from build123d import *

# Parameters (mm, degrees)
F0_W     = 152.4
F0_H     = 25.019
F0_H_2   = 0.762
F1_DEPTH = 9.525
F2_DEPTH = 2.032
F4_DEPTH = 3.175
F5_DEPTH = 9.525
F6_DEPTH = 9.525


with BuildPart() as f1:
    # F0 (on Top) → F1 (new body)
    with BuildSketch(Plane.XY):
        with Locations((35.9758849268, -12.9505327462)):
            Rectangle(F0_W, F0_H)
        with Locations((35.9758849268, 12.8304672538)):
            Rectangle(F0_W, F0_H)
        with Locations((35.9758849268, -0.0600327462)):
            Rectangle(F0_W, F0_H_2)
    extrude(amount=-F1_DEPTH)

    # F0 (on Top) → F2 (cut)
    with BuildSketch(Plane.XY):
        with Locations((35.9758849268, -0.0600327462)):
            Rectangle(F0_W, F0_H_2)
    extrude(amount=-F2_DEPTH, mode=Mode.SUBTRACT)

    # F3 (on face) → F4 (cut)
    with BuildSketch(Plane.XY):
        with BuildLine():
            Line((-30.6991150732, 18.6724672538), (-30.6991150732, 5.9724672538))
            ThreePointArc((-30.6991150732, 5.9724672538), (-29.1116150732, 4.3849672538), (-27.5241150732, 5.9724672538))
            Line((-27.5241150732, 5.9724672538), (-27.5241150732, 18.6724672538))
            ThreePointArc((-27.5241150732, 18.6724672538), (-29.1116150732, 20.2599672538), (-30.6991150732, 18.6724672538))
        make_face()
        with BuildLine():
            Line((99.4758849268, -5.9909327462), (99.4758849268, -18.6909327462))
            ThreePointArc((99.4758849268, -18.6909327462), (101.0633849268, -20.2784327462), (102.6508849268, -18.6909327462))
            Line((102.6508849268, -18.6909327462), (102.6508849268, -5.9909327462))
            ThreePointArc((102.6508849268, -5.9909327462), (101.0633849268, -4.4034327462), (99.4758849268, -5.9909327462))
        make_face()
        with BuildLine():
            Line((-30.6991150732, -5.9909327462), (-30.6991150732, -18.6909327462))
            ThreePointArc((-30.6991150732, -18.6909327462), (-29.1116150732, -20.2784327462), (-27.5241150732, -18.6909327462))
            Line((-27.5241150732, -18.6909327462), (-27.5241150732, -5.9909327462))
            ThreePointArc((-27.5241150732, -5.9909327462), (-29.1116150732, -4.4034327462), (-30.6991150732, -5.9909327462))
        make_face()
        with BuildLine():
            Line((1.8446349268, -5.9909327462), (1.8446349268, -18.6909327462))
            ThreePointArc((1.8446349268, -18.6909327462), (3.4321349268, -20.2784327462), (5.0196349268, -18.6909327462))
            Line((5.0196349268, -18.6909327462), (5.0196349268, -5.9909327462))
            ThreePointArc((5.0196349268, -5.9909327462), (3.4321349268, -4.4034327462), (1.8446349268, -5.9909327462))
        make_face()
        with BuildLine():
            Line((34.3883849268, -5.9909327462), (34.3883849268, -18.6909327462))
            ThreePointArc((34.3883849268, -18.6909327462), (35.9758849268, -20.2784327462), (37.5633849268, -18.6909327462))
            Line((37.5633849268, -18.6909327462), (37.5633849268, -5.9909327462))
            ThreePointArc((37.5633849268, -5.9909327462), (35.9758849268, -4.4034327462), (34.3883849268, -5.9909327462))
        make_face()
        with BuildLine():
            Line((66.9321349268, -5.9909327462), (66.9321349268, -18.6909327462))
            ThreePointArc((66.9321349268, -18.6909327462), (68.5196349268, -20.2784327462), (70.1071349268, -18.6909327462))
            Line((70.1071349268, -18.6909327462), (70.1071349268, -5.9909327462))
            ThreePointArc((70.1071349268, -5.9909327462), (68.5196349268, -4.4034327462), (66.9321349268, -5.9909327462))
        make_face()
        with BuildLine():
            Line((1.8446349268, 18.6724672538), (1.8446349268, 5.9724672538))
            ThreePointArc((1.8446349268, 5.9724672538), (3.4321349268, 4.3849672538), (5.0196349268, 5.9724672538))
            Line((5.0196349268, 5.9724672538), (5.0196349268, 18.6724672538))
            ThreePointArc((5.0196349268, 18.6724672538), (3.4321349268, 20.2599672538), (1.8446349268, 18.6724672538))
        make_face()
        with BuildLine():
            Line((34.3883849268, 18.6724672538), (34.3883849268, 5.9724672538))
            ThreePointArc((34.3883849268, 5.9724672538), (35.9758849268, 4.3849672538), (37.5633849268, 5.9724672538))
            Line((37.5633849268, 5.9724672538), (37.5633849268, 18.6724672538))
            ThreePointArc((37.5633849268, 18.6724672538), (35.9758849268, 20.2599672538), (34.3883849268, 18.6724672538))
        make_face()
        with BuildLine():
            Line((66.9321349268, 18.6724672538), (66.9321349268, 5.9724672538))
            ThreePointArc((66.9321349268, 5.9724672538), (68.5196349268, 4.3849672538), (70.1071349268, 5.9724672538))
            Line((70.1071349268, 5.9724672538), (70.1071349268, 18.6724672538))
            ThreePointArc((70.1071349268, 18.6724672538), (68.5196349268, 20.2599672538), (66.9321349268, 18.6724672538))
        make_face()
        with BuildLine():
            Line((99.4758849268, 18.6724672538), (99.4758849268, 5.9724672538))
            ThreePointArc((99.4758849268, 5.9724672538), (101.0633849268, 4.3849672538), (102.6508849268, 5.9724672538))
            Line((102.6508849268, 5.9724672538), (102.6508849268, 18.6724672538))
            ThreePointArc((102.6508849268, 18.6724672538), (101.0633849268, 20.2599672538), (99.4758849268, 18.6724672538))
        make_face()
    extrude(amount=-F4_DEPTH, mode=Mode.SUBTRACT)

    # F5 (add): a face of the model
    f5_faces = [f1.faces().sort_by_distance(p)[0] for p in [
        (112.1758849268, -0.0600327462, -4.7745272873),
    ]]
    extrude(f5_faces, amount=F5_DEPTH)

    # F6 (add): a face of the model
    f6_faces = [f1.faces().sort_by_distance(p)[0] for p in [
        (-40.2241150732, -0.0600327462, -4.7745272873),
    ]]
    extrude(f6_faces, amount=F6_DEPTH)


solid = f1.part
Design review of the part built by this model. Coordinates are the model's own, in mm. A direction names the side the tool comes from. Round coordinates to 2 decimals unless told otherwise and drop trailing zeros. Write each loop counter-clockwise with the first axis right and the second up, starting at its lowest first coordinate (ties: lowest second). Pieces come first, ordered by that corner, then holes. Notation, with made-up numbers: M -20,74.5 L -9,74.5 A20 cw -9,105.5 Z; hole C 26,73 d1. An arc over 180 degrees is marked long. One line per item, written item: value. Start each with the question number.
1. For faces 4 (the face through (36, -12, -3.175)), 5 (the face through (37, 25.34, -5)), list the 3-axis set-ups (+Z, -Z, +X, -X, +Y, -Y) from which the entire face can be reached by the end or side of a thin tool; tool diameter is ignored.
2. Clearance check with flat-ended pins moving along their axes: P1, Ø1.6, axis at x = -28.5, y = 14, coming from the +Z side (3 decimals); P2, Ø5, axis at x = 70, y = 4, coming from the +Z side. State where each tip first meets the part, or that it passes through.
3. To check wall thickness, follow probe 1 along X at (y, z) = (-9.5, -0.5); probe 2 along X at (y, z) = (-19, -1); probe 3 along Y at (x, z) = (-38, -0.5). State the ranges of each line that lie inside material, in increasing order. Write a range as from..to.
4. Take a section at B-B on x = -29. State the section outline as (y, z) points (1 decimal), then the cut area to 3 significant figures.
5. Draft analysis for pull direction Y (two halves, no side actions). For faces 1 (the face through (-49.749, 0, -5)), 2 (the face through (37, -25.46, -5)), 3 (the face through (5.02, 12, -2)), state which applies: pulls with the +Y half, pulls with the -Y half, needs draft (parallel to the pull), parting line crosses it, or undercut.
6. Take a section at A-A on y = 10. State the section outline as (x, z) points (3 decimals), then the cut area to 3 significant figures.
Computed:
1. face 4: +Z
1. face 5: +Z, -Z, +X, -X, +Y
2. P1: stops at z = -3.175
2. P2: stops at z = 0
3. probe 1: x = -49.75..-30.7, -27.52..1.84, 5.02..34.39, 37.56..66.93, 70.11..99.48, 102.65..121.7
3. probe 2: x = -49.75..-30.67, -27.55..1.88, 4.99..34.42, 37.53..66.96, 70.08..99.51, 102.62..121.7
3. probe 3: y = -25.46..-0.44, 0.32..25.34
4. outline: M -25.5,-9.5 L 25.3,-9.5 L 25.3,0 L 20.3,0 L 20.3,-3.2 L 4.4,-3.2 L 4.4,0 L 0.3,0 L 0.3,-2 L -0.4,-2 L -0.4,0 L -4.4,0 L -4.4,-3.2 L -20.3,-3.2 L -20.3,0 L -25.5,0 Z
4. area: 382 mm²
5. face 1: needs draft
5. face 2: pulls with the -Y half
5. face 3: undercut
6. outline: M -49.749,-9.525 L 121.701,-9.525 L 121.701,0 L 102.651,0 L 102.651,-3.175 L 99.476,-3.175 L 99.476,0 L 70.107,0 L 70.107,-3.175 L 66.932,-3.175 L 66.932,0 L 37.563,0 L 37.563,-3.175 L 34.388,-3.175 L 34.388,0 L 5.02,0 L 5.02,-3.175 L 1.845,-3.175 L 1.845,0 L -27.524,0 L -27.524,-3.175 L -30.699,-3.175 L -30.699,0 L -49.749,0 Z
6. area: 1,580 mm²
